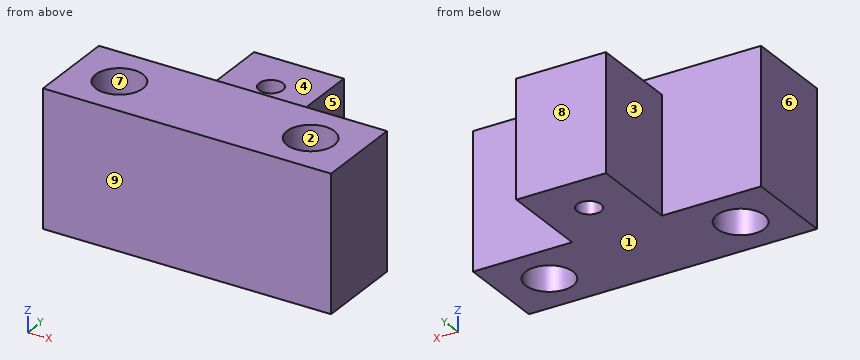
```python
from build123d import *

# Parameters (mm, degrees)
SKETCH1_R           = 0.795
BOSS_EXTRUDE1_DEPTH = 9
SKETCH4_W           = 1.25
SKETCH4_H           = 5.95656864
CUT_EXTRUDE2_DEPTH  = 13.54328432
SKETCH5_R           = 1.575
CUT_EXTRUDE3_DEPTH  = 10


with BuildPart() as part:
    # Sketch1 → Boss-Extrude1 (new body)
    with BuildSketch(Plane.XY):
        Polygon((0, 0), (0, 5.95656864), (6.58671568, 5.95656864), (6.58671568, 11.91313728), (12.54328432, 11.91313728), (12.54328432, 5.95656864), (19.13, 5.95656864), (19.13, 0), align=None)
        with Locations((9.565, 8.93485296)):
            Circle(SKETCH1_R, mode=Mode.SUBTRACT)
    extrude(amount=BOSS_EXTRUDE1_DEPTH)

    # Sketch4 → Cut-Extrude2 (cut, through all)
    with BuildSketch(Plane(origin=(12.54328432, 0, 0), x_dir=(0, 0, -1), z_dir=(1, 0, 0))):
        with Locations((-8.375, 8.93485296)):
            Rectangle(SKETCH4_W, SKETCH4_H)
    extrude(amount=-CUT_EXTRUDE2_DEPTH, mode=Mode.SUBTRACT)

    # Sketch5 → Cut-Extrude3 (cut, through all)
    with BuildSketch(Plane(origin=(0, 0, 0), x_dir=(-1, 0, 0), z_dir=(0, 0, -1))):
        with Locations((-3.215, 2.97828432)):
            Circle(SKETCH5_R)
        with Locations((-15.915, 2.97828432)):
            Circle(SKETCH5_R)
    extrude(amount=-CUT_EXTRUDE3_DEPTH, mode=Mode.SUBTRACT)


solid = part.part
```
Can you work these out from the model? Positions are in its coordinate system, mm. Face numbers are marked on the shaded views. A direction names the side the tool comes from. Coordinates: 2 decimals unless noted, no trailing zeros. Loops run counter-clockwise (first coordinate to the right, second up) from the corner with the lowest first, then second, coordinate; pieces in that order, holes last. Notation, with made-up numbers: (-6, 7) - (38, 7) arc R28 ccw to (38, 45) - close; hole circle Ø2 at (70, 23.25). An arc over 180 degrees is marked (long way). Answer as CSV lines item,"result". Start each with the question number.
1) Suppose I cut it at B-B (y = 4.25). Please give me the cut outline in (x, z), plus the area to 3 significant figures.
2) Thinking about a two-plate mould opening in Y: for the marked faces 6, 7, 8 and 9, which applies, pulls with the +Y half, pulls with the -Y half, needs draft (parallel to the pull), parting line crosses it, or undercut?
3) Which directions (+Z, -Z, +X, -X, +Y, -Y) give clear straight access to the entire face, cutting with the end or side of a thin tool? Please do the marked faces 1, 2, 3, 4 and 5.
4) I need wall thicknesses on line 1 (X direction, y = 4, z = 1.5); line 2 (X direction, y = 9, z = 6.5); line 3 (Y direction, x = 5, z = 4). Which ranges of each line are inside material? Lowest first, please. Write a range as from..to.
5) Suppose I cut it at A-A (x = 9.75). Please give me the cut outline in (y, z), plus the area to 3 significant figures.
6) Suppose I cut it at C-C (x = 7.5). Please give me the cut outline in (y, z), plus the area to 3 significant figures.
7) Suppose I cut it at D-D (z = 4). Please give me the cut outline in (x, y) (3 decimals).
8) For pin 1 (1 mm diameter, centred on y = 8, z = 6, fed in from -X); pin 2 (2.5 mm diameter, centred on x = 5, z = 2.5, fed in from +Y); pin 3 (3 mm diameter, centred on y = 10, z = 2.5, fed in from +X), each with a flat end and sliding along its axis, tell me the tip position at first contact or that it passes through.
Check result:
1,outline,"(0, 0) - (2.29, 0) - (2.29, 9) - (0, 9) - close; (4.14, 0) - (14.99, 0) - (14.99, 9) - (4.14, 9) - close; (16.84, 0) - (19.13, 0) - (19.13, 9) - (16.84, 9) - close"
1,area,"139 mm²"
2,face 6,"needs draft"
2,face 7,"undercut"
2,face 8,"pulls with the +Y half"
2,face 9,"pulls with the -Y half"
3,face 1,"-Z, +X, -X, +Y, -Y"
3,face 2,"+Z, -Z"
3,face 3,"+Z, -Z, -X, +Y"
3,face 4,"+Z, +X, -X, +Y"
3,face 5,"+Z, -Z, +X, +Y"
4,line 1,"x = 0..2.02, 4.41..14.72, 17.11..19.13"
4,line 2,"x = 6.59..8.77, 10.36..12.54"
4,line 3,"y = 0..5.96"
5,outline,"(0, 0) - (8.16, 0) - (8.16, 7.75) - (5.96, 7.75) - (5.96, 9) - (0, 9) - close; (9.71, 0) - (11.91, 0) - (11.91, 7.75) - (9.71, 7.75) - close"
5,area,"87.8 mm²"
6,outline,"(0, 0) - (11.91, 0) - (11.91, 7.75) - (5.96, 7.75) - (5.96, 9) - (0, 9) - close"
6,area,"99.8 mm²"
7,outline,"(0, 0) - (19.13, 0) - (19.13, 5.957) - (12.543, 5.957) - (12.543, 11.913) - (6.587, 11.913) - (6.587, 5.957) - (0, 5.957) - close; hole circle Ø3.15 at (3.215, 2.978); hole circle Ø1.59 at (9.565, 8.935); hole circle Ø3.15 at (15.915, 2.978)"
8,pin 1,"stops at x = 6.59"
8,pin 2,"stops at y = 5.96"
8,pin 3,"stops at x = 12.54"
